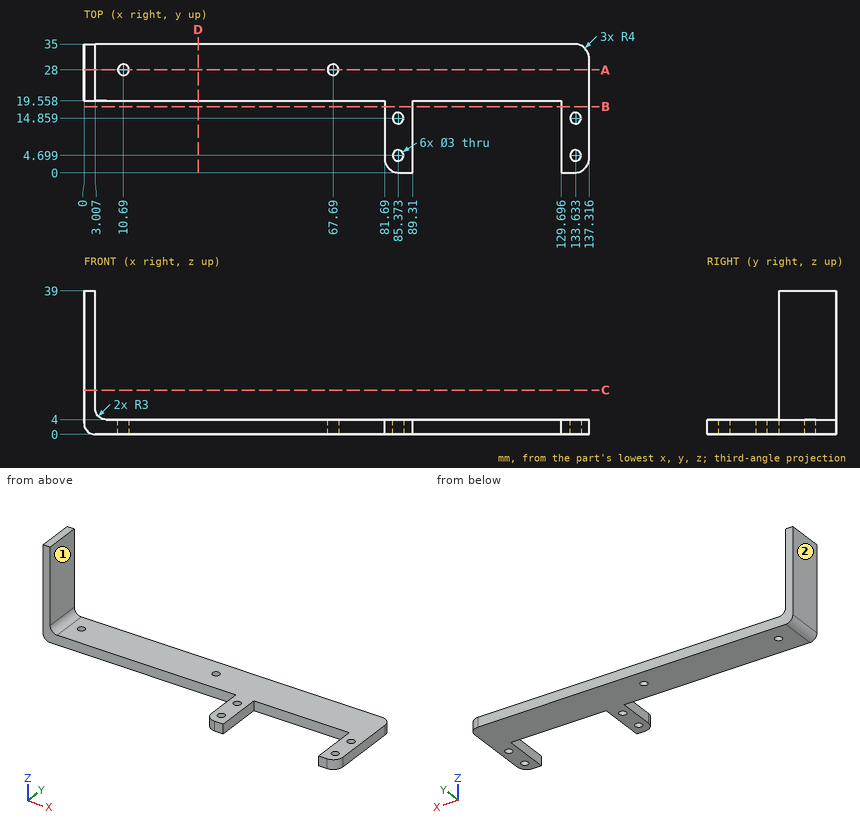
Geometry check sheet. Reference: drawing and pictorial views, mm from the part's lowest x, y, z. A direction names the side the tool comes from. Give positions to 0.01 mm unless a question says otherwise; leave off trailing zeros. Loops run counter-clockwise (first coordinate to the right, second up) from the corner with the lowest first, then second, coordinate; pieces in that order, holes last. Notation, with made-up numbers: M 61.5,52 L 118.5,52 A15 cw 118.5,59 Z; hole C 52.5,-30.5 d2. An arc over 180 degrees is marked long. One line per question, with ' | ' between items.
Item 1: Section check A-A, the plane y = 28. Record the cut outline in (x, z) (1 decimal).
Completed:
outline: M 0,3 A3 ccw 3,0 L 9.2,0 L 9.2,4 L 6,4 A3 cw 3,7 L 3,39 L 0,39 Z; M 12.2,0 L 66.2,0 L 66.2,4 L 12.2,4 Z; M 69.2,0 L 137.3,0 L 137.3,4 L 69.2,4 Z
Item 2: Section check C-C, the plane z = 12. Record the cut outline in (x, y).
Completed:
outline: M 0,19.56 L 3.01,19.56 L 3.01,35 L 0,35 Z
Item 3: Tool access check on the marked faces 1 and 2. Record the directions out of +Z, -Z, +X, -X, +Y, -Y that give a thin tool (end or side, any length) a straight path to the whole face; none if there is none.
Completed:
face 1: +Z, +X, +Y, -Y | face 2: +Z, -Z, -X, +Y, -Y
Item 4: Section check D-D, the plane x = 31. Record the cut outline in (y, z).
Completed:
outline: M 19.56,0 L 35,0 L 35,4 L 19.56,4 Z
Item 5: Depth check by flat-ended pin: P1, Ø2, axis at y = 7, z = 2, coming from the -X side; P2, Ø17, axis at y = 24, z = 29, coming from the +X side; P3, Ø1.2, axis at x = 109, z = 3, coming from the -Y side. Enter the tip coordinate at first touch or a pass-through.
Completed:
P1: stops at x = 81.69 | P2: stops at x = 3.01 | P3: stops at y = 19.56
Item 6: Section check B-B, the plane y = 18. Record the cut outline in (x, z) (1 decimal).
Completed:
outline: M 81.7,0 L 89.3,0 L 89.3,4 L 81.7,4 Z; M 129.7,0 L 137.3,0 L 137.3,4 L 129.7,4 Z
Item 7: Thickness scan on line 1 (X direction, y = 31.5, z = 36); line 2 (Y direction, x = 25.5, z = 2); line 3 (Z direction, x = 32, y = 21.5). Record the ranges inside material, lowest first. Write a range as [from, to].
Completed:
line 1: x = [0, 3.01] | line 2: y = [19.56, 35] | line 3: z = [0, 4]
